from build123d import *

# Parameters (mm, degrees)
SKETCH1_R      = 58.5
SKETCH1_R_2    = 9
EXTRUDE1_DEPTH = 0.5


with BuildPart() as part:
    # Sketch1 → Extrude1 (new body)
    with BuildSketch(Plane.XY):
        with BuildLine():
            Line((-66.728148699, -67.367918985), (-24, -79))
            Line((-24, -79), (24, -79))
            Line((24, -79), (66.889545754, -65.234577195))
            ThreePointArc((66.889545754, -65.234577195), (74.927349536, -59.427811727), (78, -50))
            Line((78, -50), (78, 50))
            ThreePointArc((78, 50), (74.927349536, 59.427811727), (66.889545754, 65.234577195))
            Line((66.889545754, 65.234577195), (24, 79))
            Line((24, 79), (-24, 79))
            Line((-24, 79), (-66.728148699, 67.367918985))
            ThreePointArc((-66.728148699, 67.367918985), (-76.302214454, 60.929165645), (-80, 50))
            Line((-80, 50), (-80, -50))
            ThreePointArc((-80, -50), (-76.302214454, -60.929165645), (-66.728148699, -67.367918985))
        make_face()
        Circle(SKETCH1_R, mode=Mode.SUBTRACT)
        with Locations((62, -50)):
            Circle(SKETCH1_R_2, mode=Mode.SUBTRACT)
        with Locations((-62, -50)):
            Circle(SKETCH1_R_2, mode=Mode.SUBTRACT)
        with Locations((62, 50)):
            Circle(SKETCH1_R_2, mode=Mode.SUBTRACT)
        with Locations((-62, 50)):
            Circle(SKETCH1_R_2, mode=Mode.SUBTRACT)
    extrude(amount=EXTRUDE1_DEPTH)


solid = part.part
Can you work these out from the model? Positions are in its coordinate system, mm. Give positions to 0.01 mm unless a question says otherwise; leave off trailing zeros. Order: outer loops, then holes, each group sorted by start corner. A loop starts at its lowest first (then second) coordinate and runs counter-clockwise, first axis right, second up. Notation, with made-up numbers: M -37,32.5 L -24,32.5 A8 cw -24,38.5 Z; hole C -25,81 d3. An arc over 180 degrees is marked long. Use a Markdown table: item, result. Add a question column.
Item 1: Suppose I cut it at A-A (y = 0). List the corners of the cut face in (x, z) for me, then the cut area to 3 significant figures.
Item 2: We'd pull the mould along Y, two halves only. Please class faces 1 (the cylindrical face through (-76.4, -60.8, 0.2)), 2 (the cylindrical face through (66.84, 57.59, 0.25)), 3 (the flat face through (-37, -52, 0)): +Y half, -Y half, draft (parallel to the pull), parting line (faces both ways), or undercut.
Item 3: Suppose I cut it at B-B (z = 0.2). List the corners of the cut face in (x, y) for me, then the cut area to 3 significant figures.
Item 4: Suppose I cut it at D-D (x = -62). List the corners of the cut face in (y, z) for me, then the cut area to 3 significant figures.
Item 5: Suppose I cut it at C-C (x = 0). List the corners of the cut face in (y, z) for me.
Item 6: If I drill on L1, parallel to Y at x = -62, z = 0.45; L2, parallel to Y at x = 62, z = 0.3; L3, parallel to X at y = -34, z = 0.1, over which ranges is the centre line in solid material (lowest first)? Write a range as [from, to].
Answer sheet:
| question | item | result |
|---|---|---|
| 1 | outline | M -80,0 L -58.5,0 L -58.5,0.5 L -80,0.5 Z; M 58.5,0 L 78,0 L 78,0.5 L 58.5,0.5 Z |
| 1 | area | 20.5 mm² |
| 2 | face 1 | -Y half |
| 2 | face 2 | undercut |
| 2 | face 3 | draft |
| 3 | outline | M -80,-50 A18 ccw -66.73,-67.37 L -24,-79 L 24,-79 L 66.89,-65.23 A16 ccw 78,-50 L 78,50 A16 ccw 66.89,65.23 L 24,79 L -24,79 L -66.73,67.37 A18 ccw -80,50 Z; hole C -62,-50 d18; hole C -62,50 d18; hole C 0,0 d117; hole C 62,-50 d18; hole C 62,50 d18 |
| 3 | area | 11,300 mm² |
| 4 | outline | M -68.66,0 L -59,0 L -59,0.5 L -68.66,0.5 Z; M -41,0 L 41,0 L 41,0.5 L -41,0.5 Z; M 59,0 L 68.66,0 L 68.66,0.5 L 59,0.5 Z |
| 4 | area | 50.7 mm² |
| 5 | outline | M -79,0 L -58.5,0 L -58.5,0.5 L -79,0.5 Z; M 58.5,0 L 79,0 L 79,0.5 L 58.5,0.5 Z |
| 6 | L1 | y = [-68.66, -59], [-41, 41], [59, 68.66] |
| 6 | L2 | y = [-66.8, -59], [-41, 41], [59, 66.8] |
| 6 | L3 | x = [-80, -47.61], [47.61, 78] |
